from build123d import *

# Parameters (mm, degrees)
F0_R     = 9.5
F0_R_2   = 5.25
F1_DEPTH = 10
F2_R     = 5.25
F2_R_2   = 3
F3_DEPTH = 5
F5_DEPTH = 12.5


with BuildPart() as f1:
    # F0 (on Top) → F1 (new body)
    with BuildSketch(Plane.XY):
        Circle(F0_R)
        Circle(F0_R_2, mode=Mode.SUBTRACT)
    extrude(amount=F1_DEPTH)

    # F2 (on Top) → F3 (join)
    with BuildSketch(Plane.XY):
        Circle(F2_R)
        Circle(F2_R_2, mode=Mode.SUBTRACT)
    extrude(amount=F3_DEPTH)

    # F4 (on Front) → F5 (intersect, symmetric)
    with BuildSketch(Plane.XZ):
        Polygon((25, 9), (-25, 10), (-25, 0), (25, 0), align=None)
    extrude(amount=F5_DEPTH, both=True, mode=Mode.INTERSECT)


solid = f1.part
For this review, take the finished solid that the model builds, in its own axes (mm). Give positions to 0.01 mm unless a question says otherwise; leave off trailing zeros. Loops run counter-clockwise (first coordinate to the right, second up) from the corner with the lowest first, then second, coordinate; pieces in that order, holes last. Notation, with made-up numbers: (-35.75, 14.5) - (-19.75, 14.5) arc R13 cw to (-19.75, 21.5) - close; hole circle Ø9 at (44.25, -12.5). An arc over 180 degrees is marked (long way). Write each question's results on one line, items separated by ' | '.
(1) For pin 1 Ø3.5 at (x, y) = (0, 0) entering from -Z; pin 2 Ø4 at (y, z) = (6, 1.5) entering from +X; pin 3 Ø1.5 at (y, z) = (-2.5, 7) entering from -X; pin 4 Ø4 at (y, z) = (3, 6.5) entering from +X, all flat-tipped, find the tip position at first contact; note any pin that passes through.
Conclusion:
pin 1: through | pin 2: x = 8.62 | pin 3: x = -9.34 | pin 4: x = 9.45
(2) Take a section at A-A (y = -0.25). Give the boundary of the cut face in (x, z), then the cut area to 3 significant figures.
Conclusion:
outline: (-9.5, 0) - (-2.99, 0) - (-2.99, 5) - (-5.24, 5) - (-5.24, 9.6) - (-9.5, 9.69) - close; (2.99, 0) - (9.5, 0) - (9.5, 9.31) - (5.24, 9.4) - (5.24, 5) - (2.99, 5) - close | area: 103 mm^2
(3) Take a section at D-D (x = -5). Give the boundary of the cut face in (y, z), then the cut area to 3 significant figures.
Conclusion:
outline: (-8.08, 0) - (8.08, 0) - (8.08, 9.6) - (1.6, 9.6) - (1.6, 5) - (-1.6, 5) - (-1.6, 9.6) - (-8.08, 9.6) - close | area: 140 mm^2
(4) Take a section at B-B (x = 0). Give the boundary of the cut face in (y, z).
Conclusion:
outline: (-9.5, 0) - (-3, 0) - (-3, 5) - (-5.25, 5) - (-5.25, 9.5) - (-9.5, 9.5) - close; (3, 0) - (9.5, 0) - (9.5, 9.5) - (5.25, 9.5) - (5.25, 5) - (3, 5) - close
(5) Draft analysis for pull direction Y (two halves, no side actions). For faces 1 (the cylindrical face through (4.38, -8.43, 4.79)), 2 (the cylindrical face through (5, 1.6, 7.3)), 3 (the cylindrical face through (-3, 0, 2)), 4 (the flat face through (-2.24, 2.24, 0)), state which applies: +Y half, -Y half, draft (parallel to the pull), parting line (faces both ways), or undercut.
Conclusion:
face 1: parting line | face 2: undercut | face 3: undercut | face 4: draft
(6) For line 1 along X through (y, z) = (0, 7.05); line 2 along Y through (x, z) = (0, 1.3), list the stretches that pass through material, from the lowest coordinate up.
Conclusion:
line 1: -9.5 to -5.25, 5.25 to 9.5 | line 2: -9.5 to -3, 3 to 9.5
(7) Take a section at C-C (z = 2.5). Give the boundary of the cut face in (x, y), then the cut area to 3 significant figures.
Conclusion:
outline: circle Ø19 at (0, 0); hole circle Ø6 at (0, 0) | area: 255 mm^2
